Part model, mm, in its own coordinate system. A direction names the side the tool comes from. Coordinates: 2 decimals unless noted, no trailing zeros. Order: outer loops, then holes, each group sorted by start corner. A loop starts at its lowest first (then second) coordinate and runs counter-clockwise, first axis right, second up.
1) Cut at C-C (x = 67.35). List the corners of the cut face in (y, z), and give its area (3 significant figures).
2) Tool access for faces 1 (the cylindrical face through (81.097, 1.141, 7.453)), 2 (the flat face through (10, 30, 7)): list every direction of +Z, -Z, +X, -X, +Y, -Y with a clear straight run to the whole face (end or side of a thin tool).
3) Mould opens along X. For faces 3 (the cylindrical face through (1.141, 1.203, 7.453)), 4 (the flat face through (24, 46, 11)), 5 (the cylindrical face through (54.29, 47.51, 12.83)), 6 (the cylindrical face through (81.159, 28.797, 7.453)) say: +X half, -X half, draft (parallel to the pull), parting line (faces both ways), or undercut.
4) Pin check, flat tips, straight feed: pin 1 Ø11.5 at (x, y) = (68, 11) entering from -Z; pin 2 Ø5 at (x, y) = (11.5, 12) entering from -Z; pin 3 Ø3.5 at (x, z) = (69.5, 10.5) entering from +Y; pin 4 Ø4 at (y, z) = (42.5, 10) entering from +X. Stop position of each tip, or through.
5) Cut at B-B (z = 8.75). Give the number of separate pieces and of enclosed holes in the cut face, and give its area (3 significant figures).
6) Cut at A-A (x = 56.65). List the corners of the cut face in (y, z), and give its area (3 significant figures).
7) Wall check: L1, parallel to Y at x = 25.65, z = 6; L2, parallel to Y at x = 56.65, z = 12; L3, parallel to X at y = 10, z = 11.5. Give the ranges that are in metal, low to high.
8) Cut at D-D (z = 1.25). List the corners of the cut face in (x, y).
```python
from build123d import *

# Parameters (mm, degrees)
SKETCH_R        = 11.3
SKETCH_R_2      = 1.6
SKETCH_R_3      = 3.2
PAD_DEPTH       = 15
SKETCH001_R     = 3.2
POCKET_DEPTH    = 4
SKETCH002_R     = 5.2
POCKET001_DEPTH = 5
FILLET_R        = 4
CHAMFER_SIZE    = 0.3
CHAMFER001_SIZE = 0.4
CHAMFER002_SIZE = 0.04


with BuildPart() as part:
    # Sketch → Pad (new body)
    with BuildSketch(Plane.XY):
        Polygon((20, 30), (20, 51), (62.3, 51), (62.3, 30), (82.3, 30), (82.3, 0), (0, 0), (0, 30), align=None)
        with Locations((41.15, 29.85)):
            Circle(SKETCH_R, mode=Mode.SUBTRACT)
        with Locations((25.65, 45.35)):
            Circle(SKETCH_R_2, mode=Mode.SUBTRACT)
        with Locations((25.65, 14.35)):
            Circle(SKETCH_R_2, mode=Mode.SUBTRACT)
        with Locations((56.65, 45.35)):
            Circle(SKETCH_R_2, mode=Mode.SUBTRACT)
        with Locations((56.65, 14.35)):
            Circle(SKETCH_R_2, mode=Mode.SUBTRACT)
        with Locations((11.15, 10)):
            Circle(SKETCH_R_3, mode=Mode.SUBTRACT)
        with Locations((67.35, 10)):
            Circle(SKETCH_R_3, mode=Mode.SUBTRACT)
        with Locations((78.75, 10)):
            Circle(SKETCH_R_3, mode=Mode.SUBTRACT)
    extrude(amount=PAD_DEPTH)

    # Sketch001 (on Face18 of Pad) → Pocket (cut)
    with BuildSketch(Plane.XY.offset(15)):
        with Locations((25.65, 45.35)):
            Circle(SKETCH001_R)
        with Locations((56.65, 45.35)):
            Circle(SKETCH001_R)
        with Locations((56.65, 14.35)):
            Circle(SKETCH001_R)
        with Locations((25.65, 14.35)):
            Circle(SKETCH001_R)
    extrude(amount=-POCKET_DEPTH, mode=Mode.SUBTRACT)

    # Sketch002 (on Face4 of Pocket) → Pocket001 (cut)
    with BuildSketch(Plane(origin=(0, 0, 0), x_dir=(1, 0, 0), z_dir=(0, 0, -1))):
        with Locations((11.15, -10)):
            Circle(SKETCH002_R)
        with Locations((67.35, -10)):
            Circle(SKETCH002_R)
        with Locations((78.75, -10)):
            Circle(SKETCH002_R)
    extrude(amount=-POCKET001_DEPTH, mode=Mode.SUBTRACT)

    # Fillet
    fillet_edges = [part.edges().sort_by_distance(p)[0] for p in [
        (82.3, 0, 7.5),
        (0, 0, 7.5),
        (0, 30, 7.5),
        (20, 30, 7.5),
        (20, 51, 7.5),
        (62.3, 51, 7.5),
        (62.3, 30, 7.5),
        (82.3, 30, 7.5),
    ]]
    fillet(fillet_edges, radius=FILLET_R)

    # Chamfer
    chamfer_edges = [part.edges().sort_by_distance(p)[0] for p in [
        (82.3, 15, 15),
        (81.128427, 1.171573, 15),
        (41.15, 0, 15),
        (1.171573, 1.171573, 15),
        (0, 15, 15),
        (1.171573, 28.828427, 15),
        (10, 30, 15),
        (18.828427, 31.171573, 15),
        (20, 40.5, 15),
        (21.171573, 49.828427, 15),
        (41.15, 51, 15),
        (61.128427, 49.828427, 15),
        (62.3, 40.5, 15),
        (63.471573, 31.171573, 15),
        (72.3, 30, 15),
        (81.128427, 28.828427, 15),
    ]]
    chamfer(chamfer_edges, length=CHAMFER_SIZE)

    # Chamfer001
    chamfer001_edges = [part.edges().sort_by_distance(p)[0] for p in [
        (64.15, 10, 15),
        (53.45, 14.35, 15),
        (22.45, 14.35, 15),
        (7.95, 10, 15),
        (22.45, 45.35, 15),
        (53.45, 45.35, 15),
    ]]
    chamfer(chamfer001_edges, length=CHAMFER001_SIZE)

    # Chamfer002
    chamfer002_edges = [part.edges().sort_by_distance(p)[0] for p in [
        (75.55, 10, 15),
    ]]
    chamfer(chamfer002_edges, length=CHAMFER002_SIZE)


solid = part.part
```
Geometry check:
1. outline: (0, 0) - (4.8, 0) - (4.8, 5) - (6.8, 5) - (6.8, 14.6) - (6.4, 15) - (0.3, 15) - (0, 14.7) - close; (13.2, 5) - (15.2, 5) - (15.2, 0) - (30, 0) - (30, 14.7) - (29.7, 15) - (13.6, 15) - (13.2, 14.6) - close
1. area: 334 mm2
2. face 1: +Z, -Z, +X, -Y
2. face 2: +Z, -Z, -X, +Y
3. face 3: -X half
3. face 4: undercut
3. face 5: undercut
3. face 6: +X half
4. pin 1: stops at z = 0
4. pin 2: stops at z = 5
4. pin 3: stops at y = 30
4. pin 4: stops at x = 62.3
5. separate pieces: 1
5. enclosed holes: 8
5. area: 2,810 mm2
6. outline: (0, 0) - (12.75, 0) - (12.75, 11) - (11.15, 11) - (11.15, 14.6) - (10.75, 15) - (0.3, 15) - (0, 14.7) - close; (15.95, 0) - (43.75, 0) - (43.75, 11) - (42.15, 11) - (42.15, 14.6) - (41.75, 15) - (17.95, 15) - (17.55, 14.6) - (17.55, 11) - (15.95, 11) - close; (46.95, 0) - (51, 0) - (51, 14.7) - (50.7, 15) - (48.95, 15) - (48.55, 14.6) - (48.55, 11) - (46.95, 11) - close
6. area: 643 mm2
7. L1: y = 0 to 12.75, 15.95 to 43.75, 46.95 to 51
7. L2: y = 0 to 11.15, 17.55 to 42.15, 48.55 to 51
7. L3: x = 0 to 7.95, 14.35 to 64.15, 70.55 to 75.55, 81.95 to 82.3
8. outline: (0, 4) arc R4 ccw to (4, 0) - (78.3, 0) arc R4 ccw to (82.3, 4) - (82.3, 6.2) arc R5.2 cw (long way) to (82.3, 13.8) - (82.3, 26) arc R4 ccw to (78.3, 30) - (66.3, 30) arc R4 cw to (62.3, 34) - (62.3, 47) arc R4 ccw to (58.3, 51) - (24, 51) arc R4 ccw to (20, 47) - (20, 34) arc R4 cw to (16, 30) - (4, 30) arc R4 ccw to (0, 26) - close; hole circle Ø10.4 at (11.15, 10); hole circle Ø3.2 at (25.65, 14.35); hole circle Ø3.2 at (25.65, 45.35); hole circle Ø22.6 at (41.15, 29.85); hole circle Ø3.2 at (56.65, 14.35); hole circle Ø3.2 at (56.65, 45.35); hole circle Ø10.4 at (67.35, 10)
